Input: part model. Units: mm. Frame: model coordinates. A direction names the side the tool comes from. Coordinates: 2 decimals unless noted, no trailing zeros. Order: outer loops, then holes, each group sorted by start corner. A loop starts at its lowest first (then second) coordinate and runs counter-clockwise, first axis right, second up. Notation, with made-up numbers: (5, 66.25) -> (60, 66.25) arc R33 ccw to (60, 97.25) -> close; hole circle Ø8 at (-36.5, -24.75). An arc over 180 degrees is marked (long way). One line per item, written item: value. Start each with the question number.
from build123d import *

# Parameters (mm, degrees)
SKETCH_1_W                       = 26
SKETCH_1_H                       = 10
SKETCH_1_R                       = 1.35
EXTRUDE_1_DEPTH                  = 1.5
SM_EDGE_FLANGE_1_STRIP_W         = 9
SM_EDGE_FLANGE_1_STRIP_H         = 1.5
SM_EDGE_FLANGE_1_STRIP_CUT_DEPTH = 26
SM_EDGE_FLANGE_1_DEPTH           = 26
SM_EDGE_FLANGE_2_STRIP_W         = 9
SM_EDGE_FLANGE_2_STRIP_H         = 1.5
SM_EDGE_FLANGE_2_STRIP_CUT_DEPTH = 26
SM_EDGE_FLANGE_2_DEPTH           = 26
SM_EDGE_FLANGE_3_STRIP_W         = 9
SM_EDGE_FLANGE_3_STRIP_H         = 1.5
SM_EDGE_FLANGE_3_STRIP_CUT_DEPTH = 26
SM_EDGE_FLANGE_3_DEPTH           = 26
SM_EDGE_FLANGE_4_STRIP_W         = 9
SM_EDGE_FLANGE_4_STRIP_H         = 1.5
SM_EDGE_FLANGE_4_STRIP_CUT_DEPTH = 26
SM_EDGE_FLANGE_4_DEPTH           = 26
SKETCH_22_R                      = 1.35
CUT_EXTRUDE_1_DEPTH              = 1.5


# Sheet-metal steps are written as plain solids
with BuildPart() as part:
    # Sketch 1 → Бобышка-Вытянуть1 (new body)
    with BuildSketch(Plane(origin=(0, 0, 0), x_dir=(1, 0, 0), z_dir=(0, 1, 0))):
        with Locations((13, 5)):
            Rectangle(SKETCH_1_W, SKETCH_1_H)
        with Locations(Location((5, 6, 0), (0, 0, 270))):
            Circle(SKETCH_1_R, mode=Mode.SUBTRACT)
        with Locations(Location((21, 6, 0), (0, 0, 270))):
            Circle(SKETCH_1_R, mode=Mode.SUBTRACT)
    extrude(amount=EXTRUDE_1_DEPTH)

    # Ребро-кромка1 strip (across the edge) → Ребро-кромка1 strip cut (cut)
    with BuildSketch(Plane(origin=(0, 1.5, 0), x_dir=(0, 0, -1), z_dir=(1, 0, 0))):
        with Locations((-1.5, -0.75)):
            Rectangle(SM_EDGE_FLANGE_1_STRIP_W, SM_EDGE_FLANGE_1_STRIP_H)
    extrude(amount=SM_EDGE_FLANGE_1_STRIP_CUT_DEPTH, mode=Mode.SUBTRACT)

    # Ребро-кромка1 section (across the edge) → Ребро-кромка1 (add)
    with BuildSketch(Plane(origin=(0, 1.5, 0), x_dir=(0, 0, -1), z_dir=(1, 0, 0))):
        with BuildLine():
            Line((0, 1.5), (0, 23))
            Line((0, 23), (1.5, 23))
            Line((1.5, 23), (1.5, 1.5))
            ThreePointArc((1.5, 1.5), (1.939339828, 0.439339828), (3, 0))
            Line((3, 0), (3, -1.5))
            ThreePointArc((3, -1.5), (0.878679656, -0.621320344), (0, 1.5))
        make_face()
    extrude(amount=SM_EDGE_FLANGE_1_DEPTH)

    # Ребро-кромка2 strip (across the edge) → Ребро-кромка2 strip cut (cut)
    with BuildSketch(Plane(origin=(26, 24.5, 0), x_dir=(0, -1, 0), z_dir=(-1, 0, 0))):
        with Locations((-1.5, -0.75)):
            Rectangle(SM_EDGE_FLANGE_2_STRIP_W, SM_EDGE_FLANGE_2_STRIP_H)
    extrude(amount=SM_EDGE_FLANGE_2_STRIP_CUT_DEPTH, mode=Mode.SUBTRACT)

    # Ребро-кромка2 section (across the edge) → Ребро-кромка2 (add)
    with BuildSketch(Plane(origin=(26, 24.5, 0), x_dir=(0, -1, 0), z_dir=(-1, 0, 0))):
        with BuildLine():
            Line((0, 1.5), (0, 45.5))
            Line((0, 45.5), (1.5, 45.5))
            Line((1.5, 45.5), (1.5, 1.5))
            ThreePointArc((1.5, 1.5), (1.939339828, 0.439339828), (3, 0))
            Line((3, 0), (3, -1.5))
            ThreePointArc((3, -1.5), (0.878679656, -0.621320344), (0, 1.5))
        make_face()
    extrude(amount=SM_EDGE_FLANGE_2_DEPTH)

    # Ребро-кромка3 strip (across the edge) → Ребро-кромка3 strip cut (cut)
    with BuildSketch(Plane(origin=(26, 23, 45.5), x_dir=(0, 0, -1), z_dir=(-1, 0, 0))):
        with Locations((-1.5, -0.75)):
            Rectangle(SM_EDGE_FLANGE_3_STRIP_W, SM_EDGE_FLANGE_3_STRIP_H)
    extrude(amount=SM_EDGE_FLANGE_3_STRIP_CUT_DEPTH, mode=Mode.SUBTRACT)

    # Ребро-кромка3 section (across the edge) → Ребро-кромка3 (add)
    with BuildSketch(Plane(origin=(26, 23, 45.5), x_dir=(0, 0, -1), z_dir=(-1, 0, 0))):
        with BuildLine():
            Line((0, 1.5), (0, 16.1))
            Line((0, 16.1), (1.5, 16.1))
            Line((1.5, 16.1), (1.5, 1.5))
            ThreePointArc((1.5, 1.5), (1.939339828, 0.439339828), (3, 0))
            Line((3, 0), (3, -1.5))
            ThreePointArc((3, -1.5), (0.878679656, -0.621320344), (0, 1.5))
        make_face()
    extrude(amount=SM_EDGE_FLANGE_3_DEPTH)

    # Ребро-кромка4 strip (across the edge) → Ребро-кромка4 strip cut (cut)
    with BuildSketch(Plane(origin=(0, 6.9, 45.5), x_dir=(0, 1, 0), z_dir=(1, 0, 0))):
        with Locations((-1.5, -0.75)):
            Rectangle(SM_EDGE_FLANGE_4_STRIP_W, SM_EDGE_FLANGE_4_STRIP_H)
    extrude(amount=SM_EDGE_FLANGE_4_STRIP_CUT_DEPTH, mode=Mode.SUBTRACT)

    # Ребро-кромка4 section (across the edge) → Ребро-кромка4 (add)
    with BuildSketch(Plane(origin=(0, 6.9, 45.5), x_dir=(0, 1, 0), z_dir=(1, 0, 0))):
        with BuildLine():
            Line((0, 1.5), (0, 18.5))
            Line((0, 18.5), (1.5, 18.5))
            Line((1.5, 18.5), (1.5, 1.5))
            ThreePointArc((1.5, 1.5), (1.939339828, 0.439339828), (3, 0))
            Line((3, 0), (3, -1.5))
            ThreePointArc((3, -1.5), (0.878679656, -0.621320344), (0, 1.5))
        make_face()
    extrude(amount=SM_EDGE_FLANGE_4_DEPTH)

    # Эскиз22 → Вырез-Вытянуть1 (cut)
    with BuildSketch(Plane(origin=(0, 8.4, 0), x_dir=(1, 0, 0), z_dir=(0, 1, 0))):
        with Locations(Location((5, -57, 0), (0, 0, 270))):
            Circle(SKETCH_22_R)
        with Locations(Location((21, -57, 0), (0, 0, 270))):
            Circle(SKETCH_22_R)
    extrude(amount=-CUT_EXTRUDE_1_DEPTH, mode=Mode.SUBTRACT)


solid = part.part
1) Section query D-D, the plane x = 7.5. Return the cut outline in (y, z).
2) Section query B-B, the plane y = 11. Return the cut outline in (x, z).
3) Section query C-C, the plane z = 57. Return the cut outline in (x, y).
4) Pin query (flat end, axial travel): pin 1 Ø8.5 at (x, z) = (10.5, 53) entering from +Y; pin 2 Ø4.5 at (x, z) = (21, -6) entering from +Y; pin 3 Ø3.5 at (x, y) = (13, 16.5) entering from -Z; pin 4 Ø2 at (x, z) = (5, -6) entering from -Y. Return the tip coordinate at first contact, or that it passes through.
5) Mould query, pull axis Z, two halves, no side actions, for faces 6 (the cylindrical face through (12.82, 7.8, 44.86)), 7 (the flat face through (13, 1, -10)), 8 (the flat face through (0, 23.2, 16.2)), 9 (the cylindrical face through (5.406, 0.74, -4.712)). Classes: +Z half, -Z half, draft (parallel to the pull), parting line (faces both ways), or undercut.
6) Ray query, line 1 along X through (y, z) = (7.85, 57); line 2 along Z through (x, y) = (15.75, 17.75); line 3 along Y through (x, z) = (8.75, 1.5). Return the intervals inside material, ascending. Write a range as from..to.
7) Section query A-A, the plane x = 21. Return the cut outline in (y, z), plus the area to 3 significant figures.
8) Access query for faces 1 (the flat face through (13, 16, 44)), 2 (the flat face through (26, 23.2, 16.2)), 3 (the cylindrical face through (19.68, 7.66, 56.71)), 4 (the flat face through (13, 1.5, -7)), 5 (the flat face through (13, 16, 45.5)). Directions: +Z, -Z, +X, -X, +Y, -Y. A direction counts if a zero-diameter tool reaches every point of the face in a straight line with its end or side. Return the directions, or none.
Entries:
1. outline: (0, -10) -> (1.5, -10) -> (1.5, -3) arc R1.5 cw to (3, -1.5) -> (21.5, -1.5) arc R3 ccw to (24.5, 1.5) -> (24.5, 42.5) arc R3 ccw to (21.5, 45.5) -> (9.9, 45.5) arc R1.5 cw to (8.4, 47) -> (8.4, 64) -> (6.9, 64) -> (6.9, 47) arc R3 ccw to (9.9, 44) -> (21.5, 44) arc R1.5 cw to (23, 42.5) -> (23, 1.5) arc R1.5 cw to (21.5, 0) -> (3, 0) arc R3 ccw to (0, -3) -> close
2. outline: (0, -1.5) -> (26, -1.5) -> (26, 0) -> (0, 0) -> close; (0, 44) -> (26, 44) -> (26, 45.5) -> (0, 45.5) -> close
3. outline: (0, 6.9) -> (3.65, 6.9) -> (3.65, 8.4) -> (0, 8.4) -> close; (6.35, 6.9) -> (19.65, 6.9) -> (19.65, 8.4) -> (6.35, 8.4) -> close; (22.35, 6.9) -> (26, 6.9) -> (26, 8.4) -> (22.35, 8.4) -> close
4. pin 1: stops at y = 8.4
4. pin 2: stops at y = 1.5
4. pin 3: stops at z = -1.5
4. pin 4: passes through
5. face 6: undercut
5. face 7: -Z half
5. face 8: draft
5. face 9: undercut
6. line 1: x = 0..3.65, 6.35..19.65, 22.35..26
6. line 2: z = -1.5..0, 44..45.5
6. line 3: y = 23..24.5
7. outline: (0, -10) -> (1.5, -10) -> (1.5, -7.35) -> (0, -7.35) -> close; (0, -4.65) -> (1.5, -4.65) -> (1.5, -3) arc R1.5 cw to (3, -1.5) -> (21.5, -1.5) arc R3 ccw to (24.5, 1.5) -> (24.5, 42.5) arc R3 ccw to (21.5, 45.5) -> (9.9, 45.5) arc R1.5 cw to (8.4, 47) -> (8.4, 55.65) -> (6.9, 55.65) -> (6.9, 47) arc R3 ccw to (9.9, 44) -> (21.5, 44) arc R1.5 cw to (23, 42.5) -> (23, 1.5) arc R1.5 cw to (21.5, 0) -> (3, 0) arc R3 ccw to (0, -3) -> close; (6.9, 58.35) -> (8.4, 58.35) -> (8.4, 64) -> (6.9, 64) -> close
7. area: 156 mm2
8. face 1: +X, -X, -Y
8. face 2: +Z, -Z, +X, +Y, -Y
8. face 3: +Y, -Y
8. face 4: -Z, +X, -X, +Y
8. face 5: +Z, +X, -X, +Y
